```python
from build123d import *

# Parameters (mm, degrees)
BOSS_EXTRUDE1_DEPTH      = 6
M3_CLEARANCE_HOLE1_D     = 3.6
M3_CLEARANCE_HOLE1_DEPTH = 6
M3_CLEARANCE_HOLE1_TIP   = 1.081549114
FILLET1_R                = 15
SKETCH4_W                = 65
SKETCH4_H                = 9
SKETCH4_W_2              = 32.5
CUT_EXTRUDE1_DEPTH       = 2
M4_CLEARANCE_HOLE1_D     = 4.8
M4_CLEARANCE_HOLE1_DEPTH = 6
M4_CLEARANCE_HOLE1_TIP   = 1.442065486
CHAMFER1_SIZE            = 2.4
BOSS_EXTRUDE2_DEPTH      = 128
SKETCH10_W               = 128
SKETCH10_H               = 68
CUT_EXTRUDE2_DEPTH       = 195.170157336


with BuildPart() as part:
    # Sketch1 → Boss-Extrude1 (new body)
    with BuildSketch(Plane.XY):
        with BuildLine():
            Line((-32.5, 95), (-32.5, -95))
            ThreePointArc((-32.5, -95), (0, -62.5), (32.5, -95))
            Line((32.5, -95), (32.5, 95))
            Line((32.5, 95), (-32.5, 95))
        make_face()
        with BuildLine():
            ThreePointArc((32.5, -95), (0, -62.5), (-32.5, -95))
            Line((-32.5, -95), (-15.5, -95))
            Line((-15.5, -95), (-15.5, -79.5))
            Line((-15.5, -79.5), (15.5, -79.5))
            Line((15.5, -79.5), (15.5, -95))
            Line((15.5, -95), (32.5, -95))
        make_face()
        with BuildLine():
            Line((-15.5, -95), (-32.5, -95))
            ThreePointArc((-32.5, -95), (0, -127.5), (32.5, -95))
            Line((32.5, -95), (15.5, -95))
            Line((15.5, -95), (15.5, -110.5))
            Line((15.5, -110.5), (-15.5, -110.5))
            Line((-15.5, -110.5), (-15.5, -95))
        make_face()
        with BuildLine():
            Line((-14, -95), (-15.5, -95))
            Line((-15.5, -95), (-15.5, -110.5))
            Line((-15.5, -110.5), (15.5, -110.5))
            Line((15.5, -110.5), (15.5, -95))
            Line((15.5, -95), (14, -95))
            ThreePointArc((14, -95), (0, -109), (-14, -95))
        make_face()
        with BuildLine():
            Line((-15.5, -79.5), (-15.5, -95))
            Line((-15.5, -95), (-14, -95))
            ThreePointArc((-14, -95), (0, -81), (14, -95))
            Line((14, -95), (15.5, -95))
            Line((15.5, -95), (15.5, -79.5))
            Line((15.5, -79.5), (-15.5, -79.5))
        make_face()
    extrude(amount=BOSS_EXTRUDE1_DEPTH)

    # M3 Clearance Hole1
    with Locations(Plane(origin=(0, 0, 0), x_dir=(-1, 0, 0), z_dir=(0, 0, -1))):
        with Locations((-15.5, -110.5), (15.5, -110.5), (15.5, -79.5), (-15.5, -79.5)):
            Hole(M3_CLEARANCE_HOLE1_D / 2, depth=M3_CLEARANCE_HOLE1_DEPTH)
            with Locations((0, 0, -(M3_CLEARANCE_HOLE1_DEPTH + M3_CLEARANCE_HOLE1_TIP / 2))):  # 118° drill point
                Cone(0, M3_CLEARANCE_HOLE1_D / 2, M3_CLEARANCE_HOLE1_TIP, mode=Mode.SUBTRACT)

    # Fillet1
    fillet1_edges = [part.edges().sort_by_distance(p)[0] for p in [
        (-32.5, 95, 3),
        (32.5, 95, 3),
    ]]
    fillet(fillet1_edges, radius=FILLET1_R)

    # Sketch4 → Cut-Extrude1 (cut)
    with BuildSketch(Plane.XY.offset(6)):
        with Locations((0, 75.5)):
            Rectangle(SKETCH4_W, SKETCH4_H)
        with Locations((-16.25, 7.5)):
            Rectangle(SKETCH4_W_2, SKETCH4_H)
        with Locations((16.25, 7.5)):
            Rectangle(SKETCH4_W_2, SKETCH4_H)
        with Locations((0, -60.5)):
            Rectangle(SKETCH4_W, SKETCH4_H)
    extrude(amount=-CUT_EXTRUDE1_DEPTH, mode=Mode.SUBTRACT)

    # M4 Clearance Hole1
    with Locations(Plane.XY.offset(4)):
        with Locations((-24.5, -60.5), (-24.5, 75.5), (24.5, 75.5), (0, 75.5), (-24.5, 7.5), (0, 7.5), (24.5, 7.5), (24.5, -60.5), (0, -60.5)):
            Hole(M4_CLEARANCE_HOLE1_D / 2, depth=M4_CLEARANCE_HOLE1_DEPTH)
            with Locations((0, 0, -(M4_CLEARANCE_HOLE1_DEPTH + M4_CLEARANCE_HOLE1_TIP / 2))):  # 118° drill point
                Cone(0, M4_CLEARANCE_HOLE1_D / 2, M4_CLEARANCE_HOLE1_TIP, mode=Mode.SUBTRACT)

    # Chamfer1
    chamfer1_edges = [part.edges().sort_by_distance(p)[0] for p in [
        (-22.1, -60.5, 0),
        (2.4, -60.5, 0),
        (26.9, -60.5, 0),
        (26.9, 7.5, 0),
        (2.4, 7.5, 0),
        (-22.1, 7.5, 0),
        (2.4, 75.5, 0),
        (26.9, 75.5, 0),
        (-22.1, 75.5, 0),
        (13.7, -79.5, 0),
        (-17.3, -79.5, 0),
        (-17.3, -110.5, 0),
        (13.7, -110.5, 0),
    ]]
    chamfer(chamfer1_edges, length=CHAMFER1_SIZE)


with BuildPart() as body_2:
    # Sketch7 → Boss-Extrude2 (new body)
    with BuildSketch(Plane(origin=(0, 0, 0), x_dir=(-1, 0, 0), z_dir=(0, 0, -1))):
        with BuildLine():
            ThreePointArc((-34.1, -95), (0, -129.1), (34.1, -95))
            Line((34.1, -95), (34.1, 80))
            Line((34.1, 80), (32.5, 80))
            Line((32.5, 80), (32.5, -95))
            ThreePointArc((32.5, -95), (0, -127.5), (-32.5, -95))
            Line((-32.5, -95), (-32.5, 80))
            Line((-32.5, 80), (-34.1, 80))
            Line((-34.1, 80), (-34.1, -95))
        make_face()
    extrude(amount=-BOSS_EXTRUDE2_DEPTH)

    # Sketch10 → Cut-Extrude2 (cut, through all)
    with BuildSketch(Plane(origin=(34.1, 0, 0), x_dir=(0, 0, -1), z_dir=(1, 0, 0))):
        with Locations((-64, 46)):
            Rectangle(SKETCH10_W, SKETCH10_H)
    extrude(amount=-CUT_EXTRUDE2_DEPTH, mode=Mode.SUBTRACT)


solid = body_2.part
```
Build history of the part. All positions in model axes, mm. A direction names the side the tool comes from. Coordinates: 2 decimals unless noted, no trailing zeros. Order: outer loops, then holes, each group sorted by start corner. A loop starts at its lowest first (then second) coordinate and runs counter-clockwise, first axis right, second up.
Item 1: Saw through at D-D on x = 0. List the corners of the cut face in (y, z).
Filled in:
outline: (-129.1, 0) - (-127.5, 0) - (-127.5, 128) - (-129.1, 128) - close
Item 2: Saw through at B-B on z = 20.5. List the corners of the cut face in (x, y).
Filled in:
outline: (-34.1, -95) arc R34.1 ccw to (34.1, -95) - (34.1, 12) - (32.5, 12) - (32.5, -95) arc R32.5 cw to (-32.5, -95) - (-32.5, 12) - (-34.1, 12) - close
Item 3: Mould opens along X. For faces 1 (the flat face through (-33, -58, 128)), 2 (the flat face through (34.1, -41, 63)), 3 (the cylindrical face through (-0.715, -127.492, 63.104)), 4 (the cylindrical face through (0.75, -129.09, 63.1)) say: released by +X, released by -X, zero draft, split by the parting line, or undercut.
Filled in:
face 1: zero draft
face 2: released by +X
face 3: undercut
face 4: split by the parting line
Item 4: Tool access for faces 5 (the flat face through (-34.1, -42, 63)), 6 (the flat face through (-32.5, -41, 63)): list every direction of +Z, -Z, +X, -X, +Y, -Y with a clear straight run to the whole face (end or side of a thin tool).
Filled in:
face 5: +Z, -Z, -X, +Y, -Y
face 6: +Z, -Z, +Y
Item 5: Drill centre lines: L1, parallel to X at y = -63, z = 25.5; L2, parallel to X at y = -106.5, z = 18; L3, parallel to Y at x = 0.5, z = 43.5. Where is each one in solid material? Low to high.
Filled in:
L1: x = -34.1 to -32.5, 32.5 to 34.1
L2: x = -32.1 to -30.4, 30.4 to 32.1
L3: y = -129.1 to -127.5
Item 6: Drop a flat-ended pin along its axis: pin 1 Ø1.5 at (x, z) = (-5.5, 77) entering from -Y. Give the stop position or say it passes through.
Filled in:
pin 1: stops at y = -128.77
Item 7: Saw through at C-C on y = -117. List the corners of the cut face in (x, z), then the cut area to 3 significant figures.
Filled in:
outline: (-26.05, 0) - (-23.92, 0) - (-23.92, 128) - (-26.05, 128) - close; (23.92, 0) - (26.05, 0) - (26.05, 128) - (23.92, 128) - close
area: 546 mm2
Item 8: Saw through at A-A on y = -25. List the corners of the cut face in (x, z), then the cut area to 3 significant figures.
Filled in:
outline: (-34.1, 0) - (-32.5, 0) - (-32.5, 128) - (-34.1, 128) - close; (32.5, 0) - (34.1, 0) - (34.1, 128) - (32.5, 128) - close
area: 410 mm2
